Part model, mm, in its own coordinate system. A direction names the side the tool comes from. Coordinates: 2 decimals unless noted, no trailing zeros. Write each loop counter-clockwise with the first axis right and the second up, starting at its lowest first coordinate (ties: lowest second). Pieces come first, ordered by that corner, then holes. Notation, with made-up numbers: (-21, 62) - (8, 62) arc R26 ccw to (8, 100) - close; hole circle Ø7 at (45, 46). An arc over 180 degrees is marked (long way). Use a Markdown table: item, result.
```python
from build123d import *

# Parameters (mm, degrees)
F0_R           = 11
F1_DEPTH       = 20
F5_D           = 9
F5_START       = 3.5000001
F5_CBORE_D     = 13
F5_CBORE_DEPTH = 9
F9_D           = 13
F9_DEPTH       = 20
F9_START       = 1.2519233
F9_TIP         = 3.9055940237


with BuildPart() as f1:
    # F0 (on Front) → F1 (new body)
    with BuildSketch(Plane.XZ):
        with BuildLine():
            ThreePointArc((-18.6153846154, -15.0769230769), (-12.3057450128, -8.6824314212), (-10, 0))
            ThreePointArc((-10, 0), (-12.3057450128, 8.6824314212), (-18.6153846154, 15.0769230769))
            ThreePointArc((-18.6153846154, 15.0769230769), (-45, 0), (-18.6153846154, -15.0769230769))
        make_face()
        with Locations((-27.5, 0)):
            Circle(F0_R, mode=Mode.SUBTRACT)
        with BuildLine():
            ThreePointArc((-18.6153846154, 15.0769230769), (-12.3057450128, 8.6824314212), (-10, 0))
            Line((-10, 0), (-10, 10))
            Line((-10, 10), (-18.6153846154, 15.0769230769))
        make_face()
        with BuildLine():
            Line((-18.6153846154, -15.0769230769), (-10, -10))
            Line((-10, -10), (-10, 0))
            ThreePointArc((-10, 0), (-12.3057450128, -8.6824314212), (-18.6153846154, -15.0769230769))
        make_face()
        Polygon((-10, -10), (10, -10), (10, 10), (-10, 10), (-10, 0), align=None)
    extrude(amount=F1_DEPTH)

    # F5 (through all)
    # its depths count from where the whole tool has entered the part; down to there all is cleared
    with Locations(Plane(origin=(-20, 0, 0), x_dir=(0, 1, 0), z_dir=(-1, 0, 0)).offset(-F5_START)):
        with Locations((-10, 0)):
            CounterBoreHole(F5_D / 2, F5_CBORE_D / 2, F5_CBORE_DEPTH)

    # F9
    # its depths count from where the whole tool has entered the part; down to there all is cleared
    with Locations(Plane(origin=(-45, 0, 0), x_dir=(0, 1, 0), z_dir=(-1, 0, 0)).offset(-F9_START)):
        with Locations((-10, 0)):
            Hole(F9_D / 2, depth=F9_DEPTH)
            with Locations((0, 0, -(F9_DEPTH + F9_TIP / 2))):  # 118° drill point
                Cone(0, F9_D / 2, F9_TIP, mode=Mode.SUBTRACT)


solid = f1.part
```
Item 1: Band-saw the part on B-B, the plane z = 0. Give the cut face in (x, y), then the cut area to 3 significant figures.
From the geometry:
| item | result |
|---|---|
| outline | (-45, -20) - (-38.5, -20) - (-38.5, -16.5) - (-45, -16.5) - close; (-45, -3.5) - (-38.5, -3.5) - (-38.5, 0) - (-45, 0) - close; (-16.5, -20) - (10, -20) - (10, -14.5) - (-7.5, -14.5) - (-7.5, -16.5) - (-16.5, -16.5) - close; (-16.5, -3.5) - (-7.5, -3.5) - (-7.5, -5.5) - (10, -5.5) - (10, 0) - (-16.5, 0) - close |
| area | 301 mm^2 |
Item 2: Drill centre lines: probe 1 along Z at (x, y) = (5.75, -10); probe 2 along Z at (x, y) = (-27.5, -9.25); probe 3 along X at (y, z) = (-1.5, -2.5). Where is each one in solid material? Low to high.
From the geometry:
| item | result |
|---|---|
| probe 1 | -10 to -4.5, 4.5 to 10 |
| probe 2 | -17.5 to -11, 11 to 17.5 |
| probe 3 | -44.82 to -38.21, -16.79 to 10 |
Item 3: Band-saw the part on C-C, the plane y = -10.25. Give the cut face in (x, z).
From the geometry:
| item | result |
|---|---|
| outline | (-43.75, -6.5) arc R17.5 ccw to (-18.62, -15.08) - (-10, -10) - (10, -10) - (10, -4.49) - (-7.5, -4.49) - (-7.5, -6.5) - (-18.62, -6.5) arc R11 cw to (-36.38, -6.5) - close; (-43.75, 6.5) - (-36.38, 6.5) arc R11 cw to (-18.62, 6.5) - (-7.5, 6.5) - (-7.5, 4.49) - (10, 4.49) - (10, 10) - (-10, 10) - (-18.62, 15.08) arc R17.5 ccw to start |
Item 4: Which spindle directions (+Z, -Z, +X, -X, +Y, -Y) get a long thin tool onto all of the face, cutting with end or side? Do faces 5 (the face through (-7.5, -11.54, -4.42)), 6 (the face through (0, -10, 10)), 7 (the face through (0, -10, -10)). Say none if no direction does.
From the geometry:
| item | result |
|---|---|
| face 5 | -X |
| face 6 | +Z, +X, +Y, -Y |
| face 7 | -Z, +X, +Y, -Y |
Item 5: Band-saw the part on D-D, the plane x = -2. Give the cut face in (y, z), then the cut area to 3 significant figures.
From the geometry:
| item | result |
|---|---|
| outline | (-20, -10) - (0, -10) - (0, 10) - (-20, 10) - close; hole circle Ø9 at (-10, 0) |
| area | 336 mm^2 |
Item 6: Band-saw the part on A-A, the plane x = -27.5. Give the cut face in (y, z).
From the geometry:
| item | result |
|---|---|
| outline | (-20, -17.5) - (0, -17.5) - (0, -11) - (-20, -11) - close; (-20, 11) - (0, 11) - (0, 17.5) - (-20, 17.5) - close |
Item 7: Drop flat-ended pins along their axis: P1, Ø6, axis at x = -30.5, y = -7.5, coming from the +Z side; P2, Ø1.5, axis at x = -11, y = -16.5, coming from the -Z side; P3, Ø4, axis at x = -12, y = -6.5, coming from the -Z side; P4, Ø6, axis at x = 0.5, y = -10.5, coming from the +Z side. Give the stop position or say it passes through.
From the geometry:
| item | result |
|---|---|
| P1 | z = 17.5 |
| P2 | z = -11.03 |
| P3 | z = -12.36 |
| P4 | z = 10 |
Item 8: Two-plate mould, pull along Z, no slides. Class faces 1 (the face through (-36.23, -9.86, -6.69)), 2 (the face through (1.373, -14.292, -1.352)), 3 (the face through (-12, -20, 0)), 4 (the face through (-14.368, -9.86, -12.574)): pulls with the +Z half, pulls with the -Z half, needs draft (parallel to the pull), parting line crosses it, or undercut.
From the geometry:
| item | result |
|---|---|
| face 1 | undercut |
| face 2 | undercut |
| face 3 | needs draft |
| face 4 | pulls with the -Z half |
